Design review of the part built by this model. Coordinates are the model's own, in mm. Face numbers are marked on the shaded views. A direction names the side the tool comes from. Round coordinates to 2 decimals unless told otherwise and drop trailing zeros. Loops run counter-clockwise (first coordinate to the right, second up) from the corner with the lowest first, then second, coordinate; pieces in that order, holes last. Notation, with made-up numbers: (39.25, 79) -> (59.25, 79) arc R9 ccw to (59.25, 96) -> close; hole circle Ø11 at (79, 5). An arc over 180 degrees is marked (long way). Answer as CSV lines item,"result". Start each with the question number.
(1) Draft analysis for pull direction Z (two halves, no side actions). For the marked faces 1, 2 and 3, state which applies: +Z half, -Z half, draft (parallel to the pull), parting line (faces both ways), or undercut.
(2) Take a section at B-B, the plane x = 120. Write out the cut boundary in (y, z), and give its area (3 significant figures).
(3) Take a section at A-A, the plane z = 7. Write out the cut boundary in (x, y), and give its area (3 significant figures).
(4) Machinability: for the marked faces 4, 5 and 6, which of the approach directions +Z, -Z, +X, -X, +Y, -Y give a long, thin tool a straight path to every point of the face, cutting with its end or side? Answer none if there is none.
(5) Take a section at D-D, the plane z = 13.25. Write out the cut boundary in (x, y), and give its area (3 significant figures).
(6) To check wall thickness, follow line 1 (Z direction, x = 118.75, y = 13.5); line 2 (X direction, y = 26, z = 10); line 3 (X direction, y = 21.5, z = 10.75). State the ranges of each line that lie inside material, in increasing order. Write a range as from..to.
(7) Take a section at C-C, the plane y = 19.5. Write out the cut boundary in (x, z), and give its area (3 significant figures).
(8) For P1, Ø2.5, axis at x = 121, y = 18.5, coming from the +Z side; P2, Ø2.5, axis at x = 121.5, y = 18.5, coming from the -Z side; P3, Ø0.7, axis at x = 122, z = 6.5, coming from the +Y side, all flat-tipped, find the tip position at first contact; note any pin that passes through.
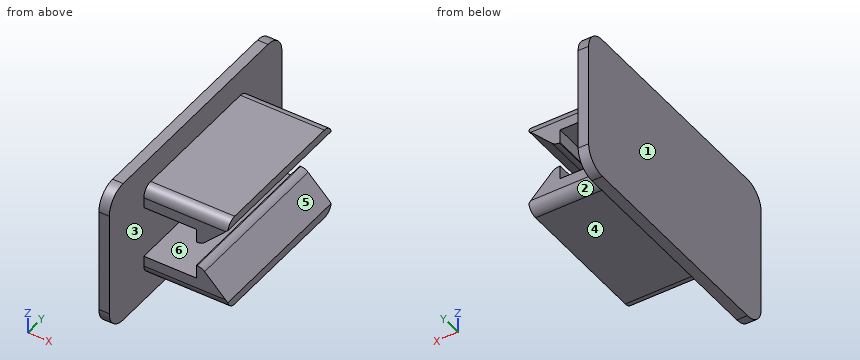
from build123d import *

# Parameters (mm, degrees)
SKETCH007_W  = 25
SKETCH007_H  = 14
PAD003_DEPTH = 1
FILLET002_R  = 2
FILLET003_R  = 2
FILLET004_R  = 2
FILLET005_R  = 2
SKETCH008_W  = 15
SKETCH008_H  = 2
PAD004_DEPTH = 5
SKETCH009_W  = 15
SKETCH009_H  = 3.3
PAD005_DEPTH = 3
CHAMFER_SIZE = 2.5
FILLET006_R  = 1
FILLET007_R  = 1
FILLET008_R  = 1


with BuildPart() as part:
    # Sketch007 → Pad003 (new body)
    with BuildSketch(Plane.YZ):
        with Locations((-12.5, 9)):
            Rectangle(SKETCH007_W, SKETCH007_H)
    extrude(amount=PAD003_DEPTH)

    # Fillet002
    fillet002_edges = [part.edges().sort_by_distance(p)[0] for p in [
        (0.5, -25, 2),
    ]]
    fillet(fillet002_edges, radius=FILLET002_R)

    # Fillet003
    fillet003_edges = [part.edges().sort_by_distance(p)[0] for p in [
        (0.5, -25, 16),
    ]]
    fillet(fillet003_edges, radius=FILLET003_R)

    # Fillet004
    fillet004_edges = [part.edges().sort_by_distance(p)[0] for p in [
        (0.5, 0, 16),
    ]]
    fillet(fillet004_edges, radius=FILLET004_R)

    # Fillet005
    fillet005_edges = [part.edges().sort_by_distance(p)[0] for p in [
        (0.5, 0, 2),
    ]]
    fillet(fillet005_edges, radius=FILLET005_R)

    # Sketch008 (on Face10 of Fillet005) → Pad004 (join)
    with BuildSketch(Plane.YZ.offset(1)):
        with Locations((-12.5, 12.5)):
            Rectangle(SKETCH008_W, SKETCH008_H)
        with Locations((-12.5, 5.5)):
            Rectangle(SKETCH008_W, SKETCH008_H)
    extrude(amount=PAD004_DEPTH)

    # Sketch009 (on Face20 of Pad004) → Pad005 (join)
    with BuildSketch(Plane.YZ.offset(6)):
        with Locations((-12.5, 6.15)):
            Rectangle(SKETCH009_W, SKETCH009_H)
        with Locations((-12.5, 11.85)):
            Rectangle(SKETCH009_W, SKETCH009_H)
    extrude(amount=PAD005_DEPTH)

    # Chamfer
    chamfer_edges = [part.edges().sort_by_distance(p)[0] for p in [
        (9, -12.5, 7.8),
        (9, -12.5, 10.2),
    ]]
    chamfer(chamfer_edges, length=CHAMFER_SIZE)

    # Fillet006
    fillet006_edges = [part.edges().sort_by_distance(p)[0] for p in [
        (6.5, -12.5, 10.2),
    ]]
    fillet(fillet006_edges, radius=FILLET006_R)

    # Fillet007
    fillet007_edges = [part.edges().sort_by_distance(p)[0] for p in [
        (6.5, -12.5, 7.8),
    ]]
    fillet(fillet007_edges, radius=FILLET007_R)

    # Fillet008
    fillet008_edges = [part.edges().sort_by_distance(p)[0] for p in [
        (3.5, -20, 4.5),
        (3.5, -20, 13.5),
        (3.5, -5, 13.5),
        (3.5, -5, 4.5),
    ]]
    fillet(fillet008_edges, radius=FILLET008_R)


with BuildPart() as part_1:
    # Body002 placement: moved
    add(part.part.moved(Location((117, 31, 0))))


solid = part_1.part
The answers:
1,face 1,"draft"
1,face 2,"-Z half"
1,face 3,"undercut"
2,outline,"(11, 5.5) arc R1 ccw to (12, 4.5) -> (25, 4.5) arc R1 ccw to (26, 5.5) -> (26, 6.5) -> (11, 6.5) -> close; (11, 11.5) -> (26, 11.5) -> (26, 12.5) arc R1 ccw to (25, 13.5) -> (12, 13.5) arc R1 ccw to (11, 12.5) -> close"
2,area,"59.1 mm²"
3,outline,"(117, 6) -> (118, 6) -> (118, 31) -> (117, 31) -> close; (123, 11) -> (124.3, 11) -> (124.3, 26) -> (123, 26) -> close"
3,area,"44.5 mm²"
4,face 4,"-Z, +X, +Y, -Y"
4,face 5,"+X, +Y, -Y"
4,face 6,"+Y, -Y"
5,outline,"(117, 6) -> (118, 6) -> (118, 11.34) -> (126, 11.34) -> (126, 25.66) -> (118, 25.66) -> (118, 31) -> (117, 31) -> close"
5,area,"140 mm²"
6,line 1,"4.5..6.5, 11.5..13.5"
6,line 2,"117..118"
6,line 3,"117..118, 123..124.05"
7,outline,"(117, 2) -> (118, 2) -> (118, 4.5) -> (126, 4.5) -> (126, 5.3) -> (123.79, 7.51) arc R1 ccw to (123.09, 7.8) -> (123, 7.8) -> (123, 6.5) -> (118, 6.5) -> (118, 11.5) -> (123, 11.5) -> (123, 10.2) -> (123.09, 10.2) arc R1 ccw to (123.79, 10.49) -> (126, 12.7) -> (126, 13.5) -> (118, 13.5) -> (118, 16) -> (117, 16) -> close"
7,area,"47.5 mm²"
8,P1,"z = 13.5"
8,P2,"z = 4.5"
8,P3,"y = 26"
